Read the model definition and answer for the solid it produces. Units are mm, in the model's axes. Face numbers are marked on the shaded views. A direction names the side the tool comes from. Round coordinates to 2 decimals unless told otherwise and drop trailing zeros. Loops run counter-clockwise (first coordinate to the right, second up) from the corner with the lowest first, then second, coordinate; pieces in that order, holes last. Notation, with made-up numbers: M -29,42 L 18,42 A13 ccw 18,63 Z; hole C 69,2 d4. An arc over 180 degrees is marked long. Answer as CSV lines item,"result".
```python
from build123d import *

# Parameters (mm, degrees)
F1_DEPTH = 76.2
F2_R     = 12.7
F3_DEPTH = 50.8


with BuildPart() as f1:
    # F0 (on Front) → F1 (new body)
    with BuildSketch(Plane.XZ):
        with BuildLine():
            Line((50.341128, 25.548994), (-51.258872, 25.548994))
            ThreePointArc((-51.258872, 25.548994), (-76.658872, 0.148994), (-51.258872, -25.251006))
            Line((-51.258872, -25.251006), (50.938825, -25.251006))
            ThreePointArc((50.938825, -25.251006), (75.742886, 0.444347), (50.341128, 25.548994))
        make_face()
    extrude(amount=F1_DEPTH)

    # F2 (on Front) → F3 (cut)
    with BuildSketch(Plane.XZ):
        with Locations((50.8, 0)):
            Circle(F2_R)
        with Locations((-50.8, 0)):
            Circle(F2_R)
    extrude(amount=F3_DEPTH, mode=Mode.SUBTRACT)


solid = f1.part
```
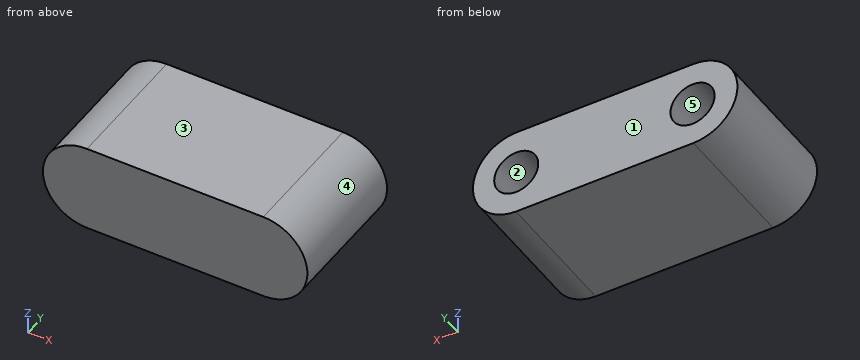
1) Each of these flat-tipped pins is pushed along its axis until it touches: P1, Ø10, axis at y = -21, z = 3.5, coming from the -X side; P2, Ø3, axis at x = -54.5, z = 4.5, coming from the +Y side; P3, Ø12, axis at x = 32, z = 5, coming from the +Y side. Where does it stop, or does it pass through?
Evaluation:
P1,"stops at x = -76.66"
P2,"stops at y = -50.8"
P3,"stops at y = 0"
2) Straight lines are drawn through the part: line 1 (Z direction, x = -50, y = -19); line 2 (Z direction, x = 61, y = -23.5); line 3 (X direction, y = -46.5, z = -8.5). For each, find the intervals that lie inside material, in ascending order.
Evaluation:
line 1,"z = -25.25 to -12.67, 12.67 to 25.55"
line 2,"z = -22.91 to -7.57, 7.57 to 23.2"
line 3,"x = -75.14 to -60.24, -41.36 to 41.36, 60.24 to 74.23"
3) Find section C-C, the plane y = -57. Give the vertices of the cut face in (x, z), then the cut area to 3 significant figures.
Evaluation:
outline,"M -51.26,-25.25 L 50.94,-25.25 A25.4 ccw 50.34,25.55 L -51.26,25.55 A25.4 ccw Z"
area,"7,190 mm^2"
4) Find section B-B, the plane z = 8. Give the vertices of the cut face in (x, y), then the cut area to 3 significant figures.
Evaluation:
outline,"M -75.42,-76.2 L 74.5,-76.2 L 74.5,0 L 60.66,0 L 60.66,-50.8 L 40.94,-50.8 L 40.94,0 L -40.94,0 L -40.94,-50.8 L -60.66,-50.8 L -60.66,0 L -75.42,0 Z"
area,"9,420 mm^2"
5) Determine the mould class of the marked faces 3, 4 and 5 for opening direction X: released by +X, released by -X, zero draft, split by the parting line, or undercut.
Evaluation:
face 3,"zero draft"
face 4,"released by +X"
face 5,"undercut"
6) A tool of negligible diameter and unlimited length cuts with its end or side. For the marked faces 1 and 2, from which of +Z, -Z, +X, -X, +Y, -Y can it reach the whole face along a straight path? Write none if from no direction.
Evaluation:
face 1,"+Z, -Z, +X, -X, +Y"
face 2,"+Y"
7) Find section A-A, the plane y = -8. Give the vertices of the cut face in (x, z).
Evaluation:
outline,"M -51.26,-25.25 L 50.94,-25.25 A25.4 ccw 50.34,25.55 L -51.26,25.55 A25.4 ccw Z; hole C -50.8,0 d25.4; hole C 50.8,0 d25.4"
8) Find section D-D, the plane z = 0. Give the vertices of the cut face in (x, y), then the cut area to 3 significant figures.
Evaluation:
outline,"M -76.66,-76.2 L 75.74,-76.2 L 75.74,0 L 63.5,0 L 63.5,-50.8 L 38.1,-50.8 L 38.1,0 L -38.1,0 L -38.1,-50.8 L -63.5,-50.8 L -63.5,0 L -76.66,0 Z"
area,"9,030 mm^2"
